```python
from build123d import *

# Parameters (mm, degrees)
SKETCH_1_W               = 40
SKETCH_1_H               = 27
EXTRUDE_1_DEPTH          = 3
EXTRUDE_2_DEPTH          = 3
SKETCH_3_W               = 40
SKETCH_3_H               = 43
EXTRUDE_3_DEPTH          = 3
SKETCH_5_R               = 11
CUT_EXTRUDE_1_DEPTH      = 59.062466362
SKETCH_6_R               = 1.6
CUT_EXTRUDE_2_DEPTH      = 59.062466362
PATTERN_CIRCULAR_1_COUNT = 4
SKETCH_7_R               = 1.6
CUT_EXTRUDE_3_DEPTH      = 69.912988616
PATTERN_LINEAR_1_COUNT   = 2
PATTERN_LINEAR_1_PITCH   = 20
MIRROR_1_COPY_1_SKETCH_R = 1.6
MIRROR_1_COPY_1_DEPTH    = 69.912988616


with BuildPart() as part:
    # 草图1 → 凸台-拉伸1 (new body)
    with BuildSketch(Plane.XY):
        Rectangle(SKETCH_1_W, SKETCH_1_H)
    extrude(amount=EXTRUDE_1_DEPTH)

    # 草图2 → 凸台-拉伸2 (add)
    with BuildSketch(Plane(origin=(0, 0, 0), x_dir=(-1, 0, 0), z_dir=(0, 0, -1))):
        with BuildLine():
            Line((-20, 13.5), (20, 13.5))
            ThreePointArc((20, 13.5), (0, 33.5), (-20, 13.5))
        make_face()
    extrude(amount=-EXTRUDE_2_DEPTH)

    # 草图3 → 凸台-拉伸3 (add)
    with BuildSketch(Plane.XZ.offset(13.5)):
        with Locations((0, 21.5)):
            Rectangle(SKETCH_3_W, SKETCH_3_H)
    extrude(amount=EXTRUDE_3_DEPTH)

    # 草图5 → 切除-拉伸1 (cut, through all)
    with BuildSketch(Plane(origin=(0, 0, 0), x_dir=(-1, 0, 0), z_dir=(0, 0, -1))):
        with Locations((0, 13.5)):
            Circle(SKETCH_5_R)
    extrude(amount=-CUT_EXTRUDE_1_DEPTH, mode=Mode.SUBTRACT)

    # 草图6 → 切除-拉伸2 (cut, through all)
    with BuildSketch(Plane(origin=(0, 0, 0), x_dir=(-1, 0, 0), z_dir=(0, 0, -1))):
        with Locations((0, 27.5)):
            Circle(SKETCH_6_R)
    cut_extrude_2 = extrude(amount=-CUT_EXTRUDE_2_DEPTH, mode=Mode.SUBTRACT)

    # 阵列(圆周)1: 切除-拉伸2 ×4 about axis
    pattern_circular_1_axis = Axis((0, 13.5, 0), (0, 0, 1))
    for i in range(1, PATTERN_CIRCULAR_1_COUNT):
        add(cut_extrude_2.rotate(pattern_circular_1_axis, i * 360 / PATTERN_CIRCULAR_1_COUNT), mode=Mode.SUBTRACT)

    # 草图7 → 切除-拉伸3 (cut, through all)
    with BuildSketch(Plane.XZ.offset(16.5)):
        with Locations((15, 33)):
            Circle(SKETCH_7_R)
    cut_extrude_3 = extrude(amount=-CUT_EXTRUDE_3_DEPTH, mode=Mode.SUBTRACT)

    # 阵列(线性)1: 切除-拉伸3 ×2
    with Locations(*[(0, 0, -i * PATTERN_LINEAR_1_PITCH) for i in range(1, PATTERN_LINEAR_1_COUNT)]):
        add(cut_extrude_3, mode=Mode.SUBTRACT)

    # 镜向1: 切除-拉伸3 across plane
    add(cut_extrude_3.mirror(Plane(origin=(0, 0, 0), x_dir=(0, 0, 1), z_dir=(1, 0, 0))), mode=Mode.SUBTRACT)

    # 镜向1 copy 1 sketch → 镜向1 copy 1 (cut, through all)
    with BuildSketch(Plane(origin=(0, -16.5, -20), x_dir=(-1, 0, 0), z_dir=(0, -1, 0))):
        with Locations((15, -33)):
            Circle(MIRROR_1_COPY_1_SKETCH_R)
    extrude(amount=-MIRROR_1_COPY_1_DEPTH, mode=Mode.SUBTRACT)


solid = part.part
```
Geometry check sheet. Reference: the model listing, model coordinates, mm. A direction names the side the tool comes from. Coordinates: 2 decimals unless noted, no trailing zeros. Order: outer loops, then holes, each group sorted by start corner. A loop starts at its lowest first (then second) coordinate and runs counter-clockwise, first axis right, second up. Notation, with made-up numbers: (19, 31) - (24, 31) arc R33 cw to (24, 64) - close; hole circle Ø1 at (-2, 61). An arc over 180 degrees is marked (long way). Use one line per item in the form item = value.
1. Draft check along X on faces 3 (the face through (-4, 0, 3)), 4 (the face through (-13.4, -15.02, 12.93)), 5 (the face through (-0.44, 33.495, 1.479)). Enter one of: pulls with the +X half, pulls with the -X half, needs draft (parallel to the pull), parting line crosses it, or undercut.
Here are the results:
face_3 = needs draft
face_4 = undercut
face_5 = parting line crosses it
2. Section check C-C (x = 6.5). Record the boundary of the cut face in (y, z), then the cut area to 3 significant figures.
Here are the results:
outline = (-16.5, 0) - (4.63, 0) - (4.63, 3) - (-13.5, 3) - (-13.5, 43) - (-16.5, 43) - close; (22.37, 0) - (32.41, 0) - (32.41, 3) - (22.37, 3) - close
area = 213 mm²
3. Section check B-B (z = 33). Record the boundary of the cut face in (x, y).
Here are the results:
outline = (-20, -16.5) - (-16.6, -16.5) - (-16.6, -13.5) - (-20, -13.5) - close; (-13.4, -16.5) - (13.4, -16.5) - (13.4, -13.5) - (-13.4, -13.5) - close; (16.6, -16.5) - (20, -16.5) - (20, -13.5) - (16.6, -13.5) - close
4. Section check D-D (x = 0). Record the boundary of the cut face in (y, z), then the cut area to 3 significant figures.
Here are the results:
outline = (-16.5, 0) - (-2.1, 0) - (-2.1, 3) - (-13.5, 3) - (-13.5, 43) - (-16.5, 43) - close; (1.1, 0) - (2.5, 0) - (2.5, 3) - (1.1, 3) - close; (24.5, 0) - (25.9, 0) - (25.9, 3) - (24.5, 3) - close; (29.1, 0) - (33.5, 0) - (33.5, 3) - (29.1, 3) - close
area = 185 mm²
5. Gauge pin test, flat ends, axial feed: pin 1 (3.5 mm diameter, centred on x = 15, z = 33, fed in from +Y); pin 2 (12 mm diameter, centred on x = 0, y = 24, fed in from +Z). Record the tip position at first contact, or that the pin passes through.
Here are the results:
pin_1 = -13.5
pin_2 = 3
6. Access from +Z, -Z, +X, -X, +Y, -Y to the whole of each face (thin tool, end or side, straight path). Record for faces 1 (the face through (20, -14, 13)), 2 (the face through (0, -13.5, 23)).
Here are the results:
face_1 = +Z, -Z, +X, +Y, -Y
face_2 = +Z, +X, -X, +Y
7. Section check A-A (y = -0.5). Record the boundary of the cut face in (x, z).
Here are the results:
outline = (-20, 0) - (-1.6, 0) - (-1.6, 3) - (-20, 3) - close; (1.6, 0) - (20, 0) - (20, 3) - (1.6, 3) - close
8. Scan lines: line 1 (Y direction, x = 0, z = 1); line 2 (Z direction, x = 15, y = -14.45); line 3 (Y direction, x = -7, z = 9). Record each from-to range of solid material in increasing order.
Here are the results:
line_1 = -16.5 to -2.1, 1.1 to 2.5, 24.5 to 25.9, 29.1 to 33.5
line_2 = 0 to 11.4, 14.6 to 31.4, 34.6 to 43
line_3 = -16.5 to -13.5
